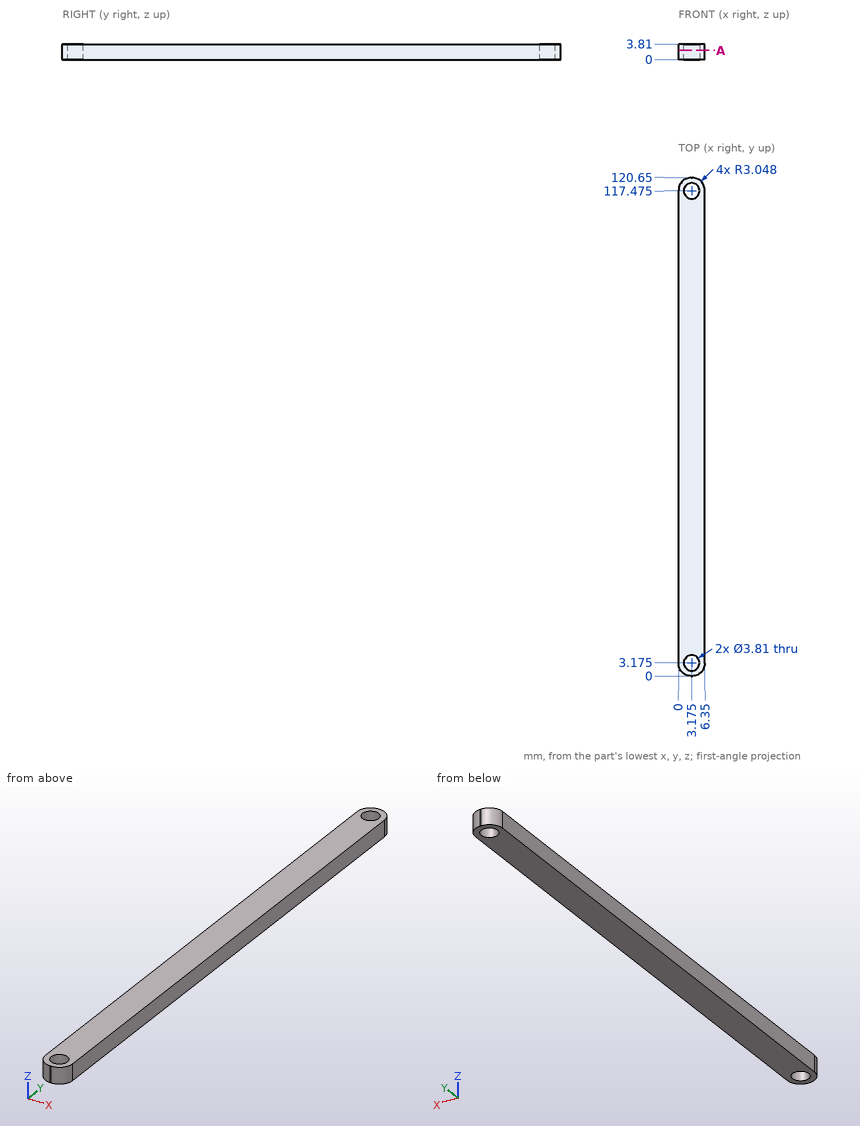
Here's the drawing with two shaded views (mm, measured from the low corner). I have some questions. Give positions to 0.01 mm unless a question says otherwise; leave off trailing zeros. Loops run counter-clockwise (first coordinate to the right, second up) from the corner with the lowest first, then second, coordinate; pieces in that order, holes last. Notation, with made-up numbers: M -34,76.5 L -1,76.5 A25 ccw -1,94.5 Z; hole C 80.5,-35 d9. An arc over 180 degrees is marked long. Answer in a Markdown table with one row per item.
1. If I drill on line 1 along Y through (x, z) = (3, 0.55); line 2 along Y through (x, z) = (1.75, 1.2); line 3 along Y through (x, z) = (5.25, 1.75), over which ranges is the centre line in solid material (lowest first)?
Taken from the geometry:
| item | result |
|---|---|
| line 1 | y = 0 to 1.28, 5.07 to 115.58, 119.37 to 120.65 |
| line 2 | y = 0.29 to 1.91, 4.44 to 116.21, 118.74 to 120.36 |
| line 3 | y = 0.7 to 119.95 |
2. For pin 1 Ø1.5 at (x, z) = (1, 2.5) entering from +Y, with a flat end and sliding along its axis, tell me the tip position at first contact or that it passes through.
Taken from the geometry:
| item | result |
|---|---|
| pin 1 | stops at y = 120.36 |
3. Suppose I cut it at A-A on z = 2.25. Write out the boundary of the cut face in (x, y) (3 decimals).
Taken from the geometry:
| item | result |
|---|---|
| outline | M 0,3.048 A3.048 ccw 3.048,0 L 3.302,0 A3.048 ccw 6.35,3.048 L 6.35,117.602 A3.048 ccw 3.302,120.65 L 3.048,120.65 A3.048 ccw 0,117.602 Z; hole C 3.175,3.175 d3.81; hole C 3.175,117.475 d3.81 |
